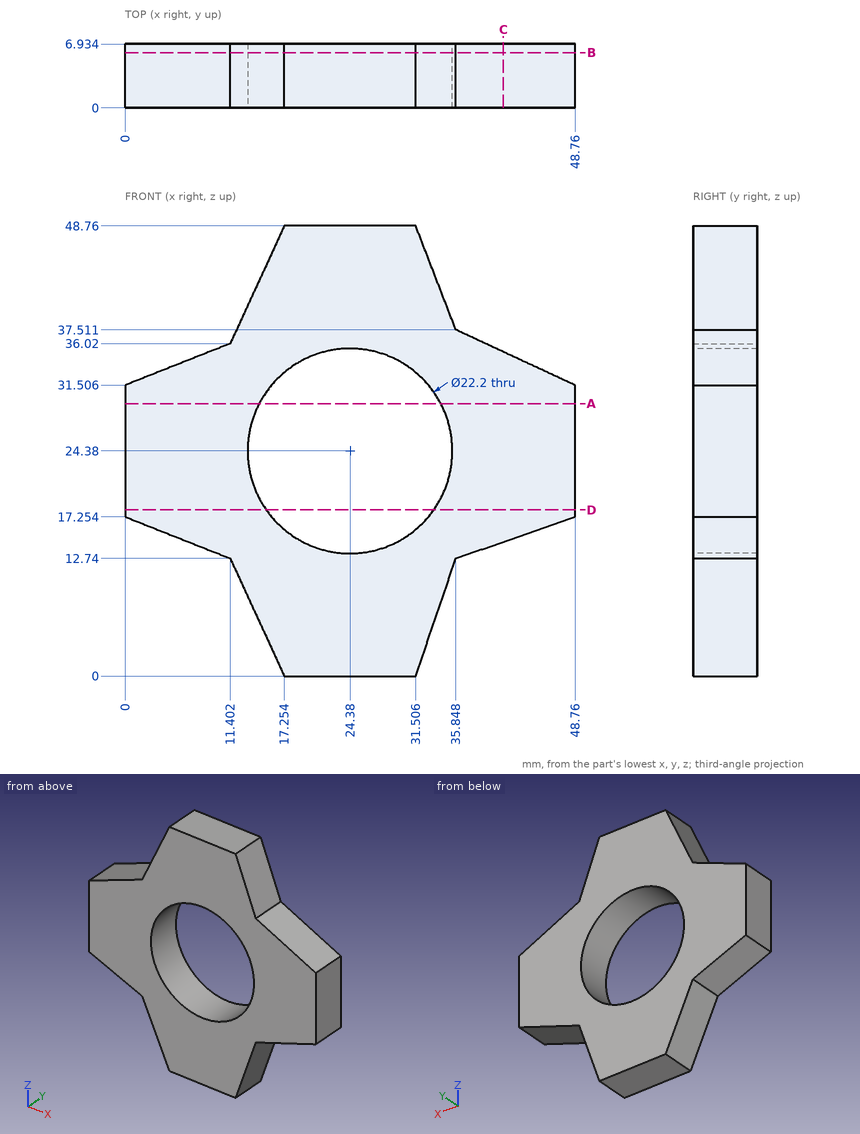
The figure shows three views and two pictorial views of one solid part (mm, origin at its lowest corner). Answer the questions. Coordinates: 2 decimals unless noted, no trailing zeros. Loops run counter-clockwise (first coordinate to the right, second up) from the corner with the lowest first, then second, coordinate; pieces in that order, holes last.
1) Find section A-A on z = 29.5. Write down the section's boundary in (x, y) (1 decimal).
2) Find section D-D on z = 18. Write down the section's boundary in (x, y) (1 decimal).
3) Find section C-C on x = 41. Write down the section's boundary in (y, z) (1 decimal), then the cut area to 3 significant figures.
4) Find the intervals of material crossed by L1, parallel to X at y = 0.5, z = 24; L2, parallel to Z at x = 27, y = 6.25 (1 decimal); L3, parallel to Z at x = 15.5, y = 6 (1 decimal), in increasing order.
5) Find section B-B on y = 6. Write down the section's boundary in (x, z) (1 decimal).
Values:
1. outline: (0, 0) - (14.5, 0) - (14.5, 6.9) - (0, 6.9) - close; (34.2, 0) - (48.8, 0) - (48.8, 6.9) - (34.2, 6.9) - close
2. outline: (0, 0) - (15.3, 0) - (15.3, 6.9) - (0, 6.9) - close; (33.5, 0) - (48.8, 0) - (48.8, 6.9) - (33.5, 6.9) - close
3. outline: (0, 14.5) - (6.9, 14.5) - (6.9, 35.1) - (0, 35.1) - close
3. area: 143 mm2
4. L1: x = 0 to 13.29, 35.47 to 48.76
4. L2: z = 0 to 13.6, 35.2 to 48.8
4. L3: z = 3.8 to 17.7, 31 to 44.9
5. outline: (0, 17.3) - (11.4, 12.7) - (17.3, 0) - (31.5, 0) - (35.8, 12.7) - (48.8, 17.3) - (48.8, 31.5) - (35.8, 37.5) - (31.5, 48.8) - (17.3, 48.8) - (11.4, 36) - (0, 31.5) - close; hole circle Ø22.2 at (24.4, 24.4)
